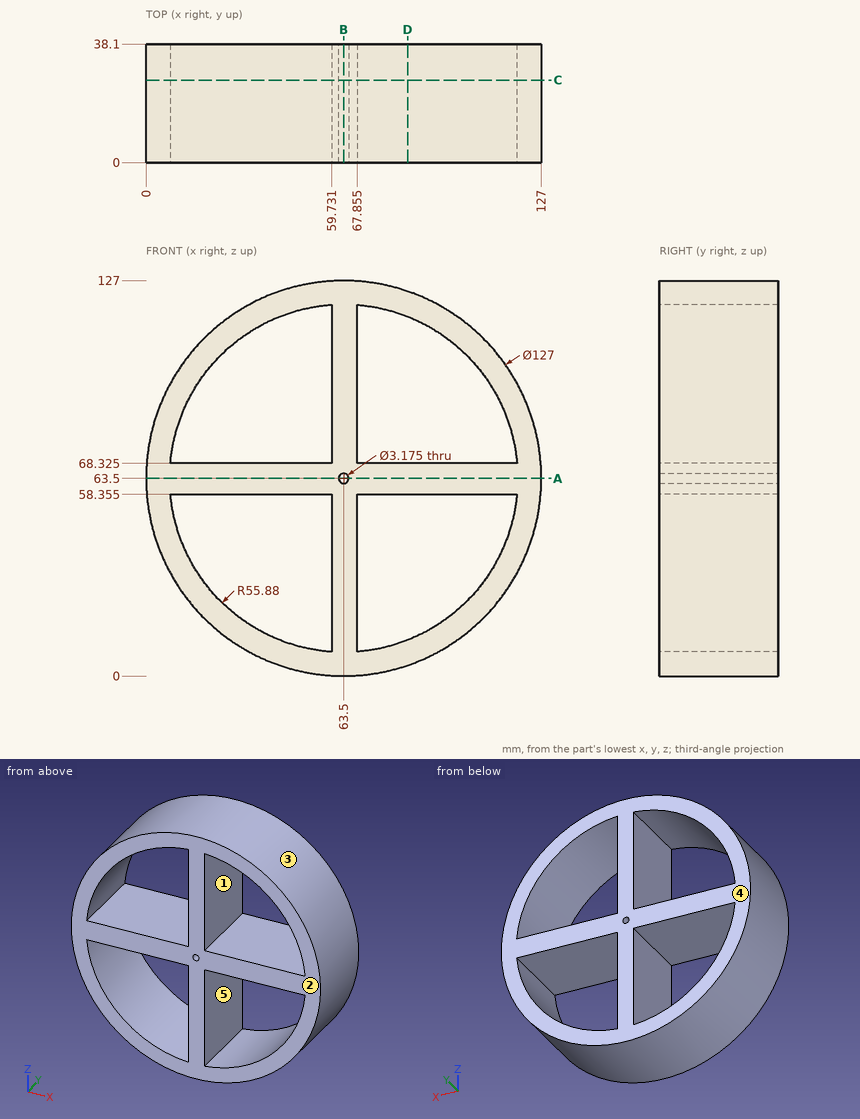
Part print with two shaded views. Sizes in mm from the minimum x, y, z corner. A direction names the side the tool comes from. Round coordinates to 2 decimals unless told otherwise and drop trailing zeros. Order: outer loops, then holes, each group sorted by start corner. A loop starts at its lowest first (then second) coordinate and runs counter-clockwise, first axis right, second up. Notation, with made-up numbers: M 88.25,37.5 L 117.25,37.5 A19 ccw 117.25,50.5 Z; hole C -29.75,28.25 d1. An arc over 180 degrees is marked long. Answer in a Markdown table with one row per item. Add a question column.
Q1. Cut at B-B on x = 63.5. Give the cut face in (y, z), and give its area (3 significant figures).
Q2. 3-axis set-ups, long thin cutter, end or side, ignore diameter. For the marked faces 4 and 5: which of +Z, -Z, +X, -X, +Y, -Y reach the whole face in a straight line?
Q3. Cut at D-D on x = 84. Give the cut face in (y, z) (1 decimal).
Q4. Cut at C-C on y = 26.5. Give the cut face in (x, z) (1 decimal), and give its area (3 significant figures).
Q5. Mould opens along X. For the marked faces 1, 2 and 3 say: +X half, -X half, draft (parallel to the pull), parting line (faces both ways), or undercut.
Q6. Pin check, flat tips, straight feed: pin 1 (5 mm diameter, centred on x = 58, z = 15, fed in from +Y); pin 2 (11.5 mm diameter, centred on x = 37, y = 20, fed in from +Z); pin 3 (12 mm diameter, centred on x = 66, y = 30, fed in from -Z); pin 4 (2 mm diameter, centred on x = 81.5, y = 7.5, fed in from +Z). Stop position of each tip, or through.
Q7. Wall check: L1, parallel to Z at x = 63.5, y = 11.5; L2, parallel to Z at x = 55, y = 6.5 (1 decimal); L3, parallel to Z at x = 110, y = 26 (1 decimal). Give the ranges that are in metal, low to high. Write a range as from..to.
Q8. Cut at A-A on z = 63.5. Give the cut face in (x, y).
Established:
| question | item | result |
|---|---|---|
| 1 | outline | M 0,0 L 38.1,0 L 38.1,61.91 L 0,61.91 Z; M 0,65.09 L 38.1,65.09 L 38.1,127 L 0,127 Z |
| 1 | area | 4,720 mm2 |
| 2 | face 4 | +Z, -Z, +X, -X, +Y |
| 2 | face 5 | +Y, -Y |
| 3 | outline | M 0,3.4 L 38.1,3.4 L 38.1,11.5 L 0,11.5 Z; M 0,58.4 L 38.1,58.4 L 38.1,68.3 L 0,68.3 Z; M 0,115.5 L 38.1,115.5 L 38.1,123.6 L 0,123.6 Z |
| 4 | outline | C 63.5,63.5 d127; hole M 7.8,68.3 L 59.7,68.3 L 59.7,119.3 A55.9 ccw Z; hole M 7.9,58.4 A55.9 ccw 59.7,7.7 L 59.7,58.4 Z; hole C 63.5,63.5 d3.2; hole M 67.9,7.8 A55.9 ccw 119.1,58.4 L 67.9,58.4 Z; hole M 67.9,68.3 L 119.2,68.3 A55.9 ccw 67.9,119.2 Z |
| 4 | area | 4,790 mm2 |
| 5 | face 1 | undercut |
| 5 | face 2 | draft |
| 5 | face 3 | parting line |
| 6 | pin 1 | stops at y = 38.1 |
| 6 | pin 2 | stops at z = 123.51 |
| 6 | pin 3 | stops at z = 0 |
| 6 | pin 4 | stops at z = 124.68 |
| 7 | L1 | z = 0..61.91, 65.09..127 |
| 7 | L2 | z = 0.6..8.3, 58.4..68.3, 118.7..126.4 |
| 7 | L3 | z = 20.3..32.5, 58.4..68.3, 94.5..106.7 |
| 8 | outline | M 0,0 L 61.91,0 L 61.91,38.1 L 0,38.1 Z; M 65.09,0 L 127,0 L 127,38.1 L 65.09,38.1 Z |
